CAD build for the part. Positions are in the model's coordinates, mm. Face numbers are marked on the shaded views. A direction names the side the tool comes from. Round coordinates to 2 decimals unless told otherwise and drop trailing zeros. Order: outer loops, then holes, each group sorted by start corner. A loop starts at its lowest first (then second) coordinate and runs counter-clockwise, first axis right, second up. Notation, with made-up numbers: (-14.5, 62) - (16.5, 62) arc R18 cw to (16.5, 66) - close; hole circle Ø9 at (-7.5, 78). An arc over 180 degrees is marked (long way). Write item = value, one per line.
Autodesk Inventor part; units mm, degrees
ref_plane "YZ Plane" through (0, 0, 0) normal (1, 0, 0) x (0, 1, 0)
ref_plane "XZ Plane" through (0, 0, 0) normal (0, 1, 0) x (-1, 0, 0)
ref_plane "XY Plane" through (0, 0, 0) normal (0, 0, 1) x (1, 0, 0)
sketch "Sketch2" plane through (0, 0, 0) normal (0, 1, 0) x (-1, 0, 0)
  circle A0 centre (0, 0) radius 2.45
  circle A1 centre (0, 6.2) radius 5.65
  line L0 (9, -9.2) -> (-9, -9.2)
  line L1 (-9, -9.2) -> (-9, 11.1)
  line L2 (-9, 11.1) -> (9, 11.1)
  line L3 (9, 11.1) -> (9, -9.2)
  circle A2 centre (6, -6.7) radius 1.4
  line L4 (0, 0) -> (0, -9.2) construction
  circle A3 centre (-6, -6.7) radius 1.4
  point P0 (2.8129, 11.1)
  point P1 (2.2323, 1.0097)
  point P2 (-2.2323, 1.0097)
  point P3 (-2.8129, 11.1)
  dimension "d20" = 4.9
  dimension "d21" = 11.3
  dimension "d22" = 6.2
  dimension "d23" = 4.9
  dimension "d24" = 18
  dimension "d25" = 20.3
  dimension "d26" = 2.8
  dimension "d27" = 2.5
  dimension "d28" = 3
extrude "Extrusion1" add sketch "Sketch2" along normal blind 3 contours A0 A1 L2 L3 L0 L1
fillet "Fillet1" radius 2.5 2 edges at (-2.2323, 1.5, 1.0097) (2.2323, 1.5, 1.0097)
properties part number "sujetador_cremallera"
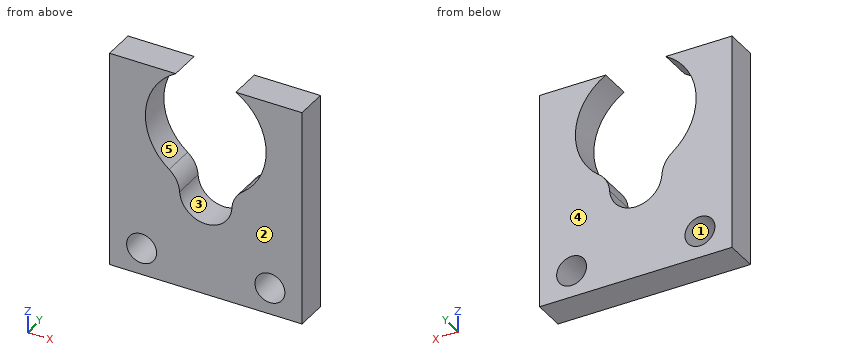
(1) Band-saw the part on D-D on y = 0.7. Count the separate pieces of the cut face and the enclosed holes in it, plus the area to 3 significant figures.
Solved:
separate_pieces = 1
enclosed_holes = 2
area = 242 mm²
(2) Band-saw the part on A-A on z = -6.7. List the corners of the cut face in (x, y).
Solved:
outline = (-9, 0) - (-7.4, 0) - (-7.4, 3) - (-9, 3) - close; (-4.6, 0) - (4.6, 0) - (4.6, 3) - (-4.6, 3) - close; (7.4, 0) - (9, 0) - (9, 3) - (7.4, 3) - close
(3) Band-saw the part on C-C on z = 8. List the corners of the cut face in (x, y).
Solved:
outline = (-9, 0) - (-5.36, 0) - (-5.36, 3) - (-9, 3) - close; (5.36, 0) - (9, 0) - (9, 3) - (5.36, 3) - close
(4) Drop a flat-ended pin along its axis: pin 1 (1 mm diameter, centred on x = -6, z = 8, fed in from -Y). Give the stop position or say it passes through.
Solved:
pin_1 = 0
(5) Band-saw the part on B-B on x = -6. List the corners of the cut face in (y, z).
Solved:
outline = (0, -9.2) - (3, -9.2) - (3, -8.1) - (0, -8.1) - close; (0, -5.3) - (3, -5.3) - (3, 11.1) - (0, 11.1) - close
(6) Pull direction Z, two halves, no side cores. Call the marked faces 1, 2 and 3: released by +Z, released by -Z, zero draft, split by the parting line, or undercut.
Solved:
face_1 = undercut
face_2 = zero draft
face_3 = released by +Z
(7) Tool access for the marked faces 4 and 5: list every direction of +Z, -Z, +X, -X, +Y, -Y with a clear straight run to the whole face (end or side of a thin tool).
Solved:
face_4 = +Z, -Z, +X, -X, +Y
face_5 = +Y, -Y
(8) Probe line 1 along Z through (x, y) = (-6, 2.3); line 2 along X through (y, z) = (2.15, -7); line 3 along X through (y, z) = (1.5, 7.5). List the from-to ranges inside material, lowest first.
Solved:
line_1 = -9.2 to -8.1, -5.3 to 11.1
line_2 = -9 to -7.37, -4.63 to 4.63, 7.37 to 9
line_3 = -9 to -5.5, 5.5 to 9
